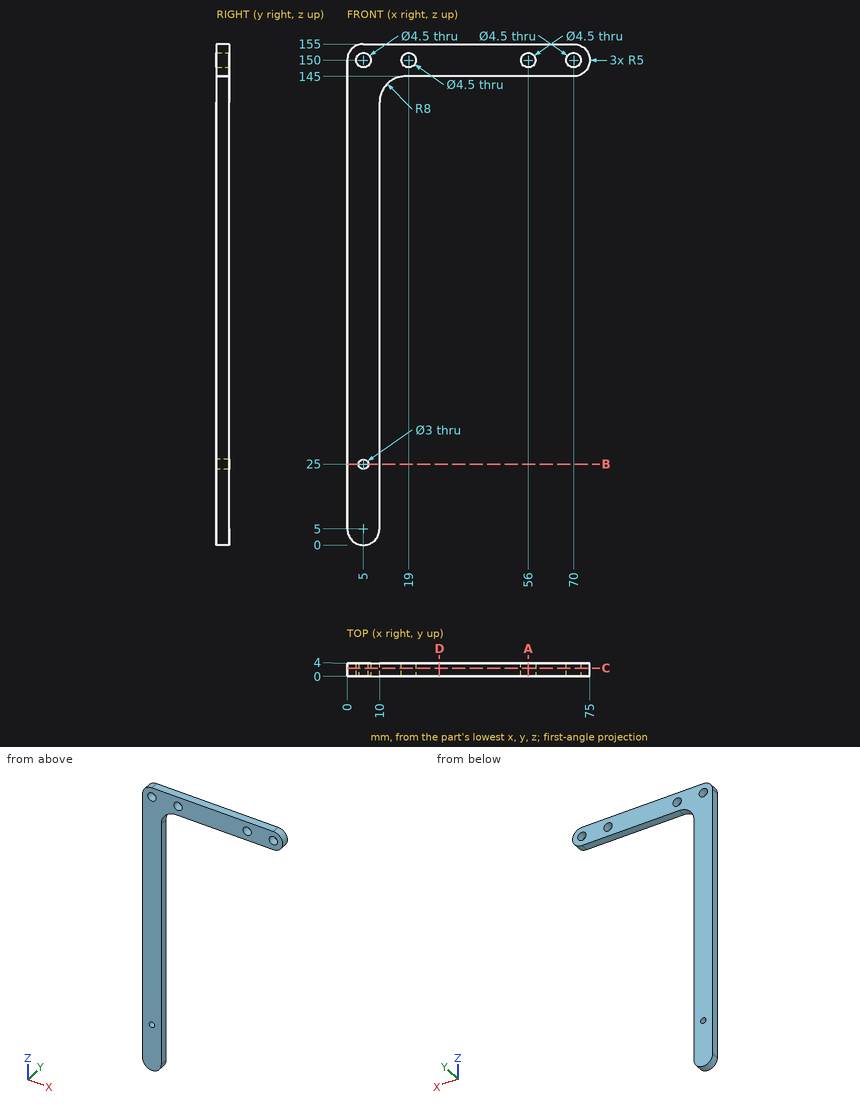
Can you work these out from the drawing? Everything is in mm from the part's minimum corner. Give positions to 0.01 mm unless a question says otherwise; leave off trailing zeros. Loops run counter-clockwise (first coordinate to the right, second up) from the corner with the lowest first, then second, coordinate; pieces in that order, holes last. Notation, with made-up numbers: (-32, -7.75) - (10, -7.75) arc R36 ccw to (10, 31.25) - close; hole circle Ø8 at (40.5, -5). An arc over 180 degrees is marked (long way). Answer as a JSON object with one key per item and string values.
Q1. Imagine slicing it at D-D on x = 28.5. Write out the boundary of the cut face in (y, z).
Geometry says:
{"outline": "(0, 145) - (4, 145) - (4, 155) - (0, 155) - close"}
Q2. Imagine slicing it at A-A on x = 56. Write out the boundary of the cut face in (y, z).
Geometry says:
{"outline": "(0, 145) - (4, 145) - (4, 147.75) - (0, 147.75) - close; (0, 152.25) - (4, 152.25) - (4, 155) - (0, 155) - close"}
Q3. If I drill on L1, parallel to X at y = 1, z = 150; L2, parallel to Z at x = 5, y = 0.95; L3, parallel to Z at x = 19, y = 2.4, over which ranges is the centre line in solid material (lowest first)?
Geometry says:
{"L1": "0 to 2.75, 7.25 to 16.75, 21.25 to 53.75, 58.25 to 67.75, 72.25 to 75", "L2": "0 to 23.5, 26.5 to 147.75, 152.25 to 155", "L3": "145 to 147.75, 152.25 to 155"}
Q4. Will these pins go through, and if not, where does the flat tip stop? P1, Ø5, axis at x = 5, z = 150, coming from the -Y side; P2, Ø1, axis at y = 2, z = 34.5, coming from the +X side.
Geometry says:
{"P1": "y = 0", "P2": "x = 10"}
Q5. Imagine slicing it at B-B on z = 25. Write out the boundary of the cut face in (x, y), plus the area to 3 significant figures.
Geometry says:
{"outline": "(0, 0) - (3.5, 0) - (3.5, 4) - (0, 4) - close; (6.5, 0) - (10, 0) - (10, 4) - (6.5, 4) - close", "area": "28.0 mm²"}
Q6. Imagine slicing it at C-C on y = 2.45. Write out the boundary of the cut face in (x, z).
Geometry says:
{"outline": "(0, 5) arc R5 ccw to (10, 5) - (10, 137) arc R8 cw to (18, 145) - (70, 145) arc R5 ccw to (70, 155) - (5, 155) arc R5 ccw to (0, 150) - close; hole circle Ø4.5 at (5, 150); hole circle Ø3 at (5, 25); hole circle Ø4.5 at (19, 150); hole circle Ø4.5 at (56, 150); hole circle Ø4.5 at (70, 150)"}
